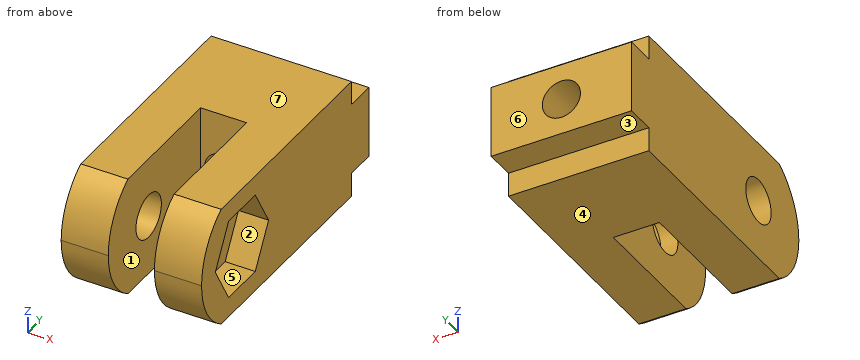
from build123d import *

# Parameters (mm, degrees)
BOSS_EXTRUDE1_DEPTH = 6
SKETCH2_R           = 1.1
CUT_EXTRUDE1_DEPTH  = 28.586228448
CUT_EXTRUDE2_DEPTH  = 1.5
SKETCH4_W           = 7
SKETCH4_H           = 3.6
BOSS_EXTRUDE2_DEPTH = 1.5
SKETCH5_R           = 0.95
CUT_EXTRUDE3_DEPTH  = 6.5


with BuildPart() as part:
    # Sketch1 → Boss-Extrude1 (new body)
    with BuildSketch(Plane.XY):
        Polygon((-1.15, 13), (-1.15, 21), (1.15, 21), (1.15, 13), (3.5, 13), (3.5, 26), (-3.5, 26), (-3.5, 13), align=None)
    extrude(amount=-BOSS_EXTRUDE1_DEPTH)

    # Sketch2 → Cut-Extrude1 (cut, through all)
    with BuildSketch(Plane(origin=(3.5, 0, 0), x_dir=(0, 0, -1), z_dir=(1, 0, 0))):
        with Locations(Location((3, 16.5, 0), (0, 0, 90))):
            Circle(SKETCH2_R)
        with BuildLine():
            ThreePointArc((3.000000016, 13), (1.276589831, 13.453714165), (0, 14.697224362))
            Line((0, 14.697224362), (0, 13))
            Line((0, 13), (3.000000016, 13))
        make_face()
        with BuildLine():
            ThreePointArc((6, 14.697224362), (4.723410183, 13.453714173), (3.000000016, 13))
            Line((3.000000016, 13), (6, 13))
            Line((6, 13), (6, 14.697224362))
        make_face()
    extrude(amount=-CUT_EXTRUDE1_DEPTH, mode=Mode.SUBTRACT)

    # Sketch3 → Cut-Extrude2 (cut)
    with BuildSketch(Plane(origin=(3.5, 0, 0), x_dir=(0, 0, -1), z_dir=(1, 0, 0))):
        Polygon((3, 18.809401077), (1, 17.654700538), (1, 15.345299462), (3, 14.190598923), (5, 15.345299462), (5, 17.654700538), align=None)
    extrude(amount=-CUT_EXTRUDE2_DEPTH, mode=Mode.SUBTRACT)

    # Sketch4 → Boss-Extrude2 (add)
    with BuildSketch(Plane(origin=(0, 26, 0), x_dir=(1, 0, 0), z_dir=(0, 1, 0))):
        with Locations((0, 3)):
            Rectangle(SKETCH4_W, SKETCH4_H)
    extrude(amount=BOSS_EXTRUDE2_DEPTH)

    # Sketch5 → Cut-Extrude3 (cut)
    with BuildSketch(Plane(origin=(0, 27.5, 0), x_dir=(1, 0, 0), z_dir=(0, 1, 0))):
        with Locations(Location((0, 3, 0), (0, 0, 270))):
            Circle(SKETCH5_R)
    extrude(amount=-CUT_EXTRUDE3_DEPTH, mode=Mode.SUBTRACT)


solid = part.part
Here's how the part is built. I have some questions about the finished solid (model axes, mm). Face numbers are marked on the shaded views. A direction names the side the tool comes from. Give positions to 0.01 mm unless a question says otherwise; leave off trailing zeros. Loops run counter-clockwise (first coordinate to the right, second up) from the corner with the lowest first, then second, coordinate; pieces in that order, holes last. Notation, with made-up numbers: (-12.75, 57.25) -> (23.25, 57.25) arc R8 cw to (23.25, 66.25) -> close; hole circle Ø3 at (-38, -27.75). An arc over 180 degrees is marked (long way). One line per item, written item: value.
Q1. We'd pull the mould along Z, two halves only. Please class the marked faces 5, 6 and 7: pulls with the +Z half, pulls with the -Z half, needs draft (parallel to the pull), parting line crosses it, or undercut.
Answers follow:
face 5: undercut
face 6: needs draft
face 7: pulls with the +Z half
Q2. Suppose I cut it at C-C on y = 16.5. Please give me the cut outline in (x, z), then the cut area to 3 significant figures.
Answers follow:
outline: (-3.5, -6) -> (-1.15, -6) -> (-1.15, -4.1) -> (-3.5, -4.1) -> close; (-3.5, -1.9) -> (-1.15, -1.9) -> (-1.15, 0) -> (-3.5, 0) -> close; (1.15, -6) -> (3.5, -6) -> (3.5, -5) -> (2, -5) -> (2, -4.1) -> (1.15, -4.1) -> close; (1.15, -1.9) -> (2, -1.9) -> (2, -1) -> (3.5, -1) -> (3.5, 0) -> (1.15, 0) -> close
area: 15.2 mm^2
Q3. Suppose I cut it at A-A on y = 19.25. Please give me the cut outline in (x, z), then the cut area to 3 significant figures.
Answers follow:
outline: (-3.5, -6) -> (-1.15, -6) -> (-1.15, 0) -> (-3.5, 0) -> close; (1.15, -6) -> (3.5, -6) -> (3.5, 0) -> (1.15, 0) -> close
area: 28.2 mm^2
Q4. I'm going to push flat-ended pins straight in: pin 1 Ø2 at (x, z) = (-1, -5) entering from -Y; pin 2 Ø1.6 at (x, y) = (0, 27) entering from +Z; pin 3 Ø0.7 at (x, z) = (-0.5, -2) entering from -Y. Where does each tip first touch, or does it pass through?
Answers follow:
pin 1: y = 13.15
pin 2: z = -1.2
pin 3: y = 21
Q5. If I drill on line 1 along Z through (x, y) = (-2.3, 16.5); line 2 along X through (y, z) = (17, -1.75); line 3 along Y through (x, z) = (1, -3.5), over which ranges is the centre line in solid material (lowest first)?
Answers follow:
line 1: -6 to -4.1, -1.9 to 0
line 2: -3.5 to -1.15, 1.15 to 2
line 3: 21 to 27.5
Q6. Suppose I cut it at D-D on x = 0. Please give me the cut outline in (y, z).
Answers follow:
outline: (21, -6) -> (26, -6) -> (26, -4.8) -> (27.5, -4.8) -> (27.5, -3.95) -> (21, -3.95) -> close; (21, -2.05) -> (27.5, -2.05) -> (27.5, -1.2) -> (26, -1.2) -> (26, 0) -> (21, 0) -> close
Q7. On a 3-axis mill with a long thin cutter (end or side, diameter ignored), from which of +Z, -Z, +X, -X, +Y, -Y can I reach the whole of each face in a straight line? I mean the marked faces 1, 2, 3 and 4. Say none if no direction works.
Answers follow:
face 1: +Z, -Z, -Y
face 2: +X
face 3: -Z, +X, -X, +Y
face 4: -Z, +X, -X, +Y, -Y
Q8. Suppose I cut it at B-B on x = 3.25. Please give me the cut outline in (y, z), then the cut area to 3 significant figures.
Answers follow:
outline: (14.7, -6) -> (26, -6) -> (26, -4.8) -> (27.5, -4.8) -> (27.5, -1.2) -> (26, -1.2) -> (26, 0) -> (14.7, 0) arc R3.5 ccw to start; hole (14.19, -3) -> (15.35, -5) -> (17.65, -5) -> (18.81, -3) -> (17.65, -1) -> (15.35, -1) -> close
area: 66.6 mm^2
